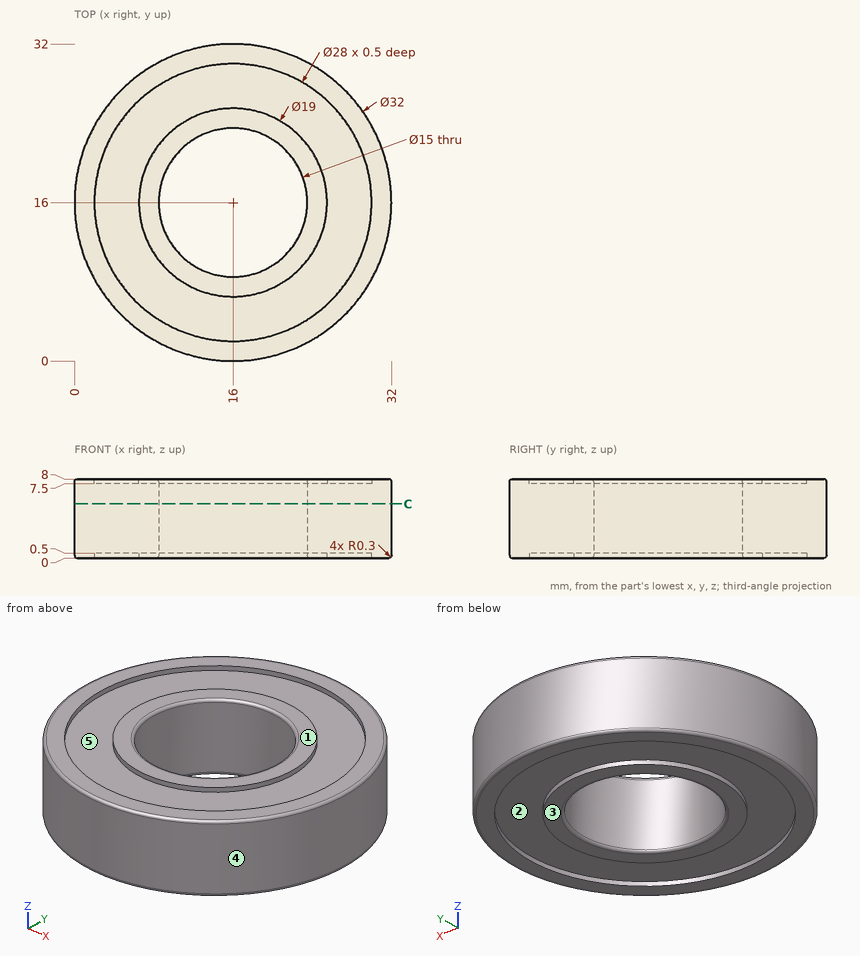
Check sheet for the drawn part. Datum: minimum x, y, z corner. Units: mm. A direction names the side the tool comes from. Round coordinates to 2 decimals unless told otherwise and drop trailing zeros. Loops run counter-clockwise (first coordinate to the right, second up) from the corner with the lowest first, then second, coordinate; pieces in that order, holes last. Notation, with made-up numbers: M 72,0 L 119,0 A18 cw 119,7 Z; hole C -27.75,58 d11. An arc over 180 degrees is marked long. Write each question's results on one line, items separated by ' | '.
1) Access from +Z, -Z, +X, -X, +Y, -Y to the whole of each face (thin tool, end or side, straight path). Record for the marked faces 1 and 2.
Checks:
face 1: +Z, +X, -X, +Y, -Y | face 2: -Z
2) Scan lines: L1, parallel to Y at x = 16, z = 0.4; L2, parallel to Y at x = 16, z = 4.5; L3, parallel to Y at x = 16, z = 0.1. Record each from-to range of solid material in increasing order. Write a range as from..to.
Checks:
L1: y = 0..2, 6.5..8.5, 23.5..25.5, 30..32 | L2: y = 0..8.5, 23.5..32 | L3: y = 0.08..2, 6.5..8.42, 23.58..25.5, 30..31.92
3) Section check C-C on z = 5.5. Record the boundary of the cut face in (x, y), then the cut area to 3 significant figures.
Checks:
outline: C 16,16 d32; hole C 16,16 d15 | area: 628 mm2
4) Gauge pin test, flat ends, axial feed: P1, Ø3, axis at x = 14, y = 27, coming from the +Z side; P2, Ø2, axis at y = 22.5, z = 2, coming from the +X side (3 decimals); P3, Ø2, axis at y = 22, z = 4.5, coming from the -X side. Record the tip position at first contact, or that the pin passes through.
Checks:
P1: stops at z = 7.5 | P2: stops at x = 31.025 | P3: stops at x = 0.8
5) Mould release check, pull along X, two halves, no side actions. Record for the marked faces 3, 4 and 5: released by +X, released by -X, zero draft, split by the parting line, or undercut.
Checks:
face 3: zero draft | face 4: split by the parting line | face 5: undercut
